Input: dimensioned drawing with shaded views. Units: mm. Origin: part minimum x, y, z. A direction names the side the tool comes from. Round coordinates to 2 decimals unless told otherwise and drop trailing zeros. Order: outer loops, then holes, each group sorted by start corner. A loop starts at its lowest first (then second) coordinate and runs counter-clockwise, first axis right, second up. Notation, with made-up numbers: M 26.5,1.25 L 39.5,1.25 A9 ccw 39.5,9.25 Z; hole C -27.75,11 d8. An arc over 180 degrees is marked long. Put each result on its own line as item: value. Start each with the question number.
1) Access query for the marked faces 1, 2 and 3. Directions: +Z, -Z, +X, -X, +Y, -Y. A direction counts if a zero-diameter tool reaches every point of the face in a straight line with its end or side. Return the directions, or none.
2) Material intervals for probe 1 along X at (y, z) = (2.25, 0.85); probe 2 along X at (y, z) = (3.5, 2.1); probe 3 along Y at (x, z) = (13.5, 0.95), sorted ascending. Write a range as [from, to].
3) First-contact query: P1, Ø1.5, axis at x = 39, z = 2, coming from the +Y side; P2, Ø1.5, axis at x = 40, y = 5, coming from the +Z side; P3, Ø1, axis at y = 13, z = 1.5, coming from the +X side; P4, Ø1, axis at y = 8.5, z = 2.5, coming from the +X side. Flat tips, straight axial feed; report the tip coordinate or a pass-through.
4) Section B-B, the plane x = 42. Return loops of the section in (y, z).
5) Section D-D, the plane x = 24.5. Return loops of the section in (y, z).
6) Section A-A, the plane y = 1.5. Return loops of the section in (x, z), then the cut area to 3 significant figures.
7) Section C-C, the plane y = 13. Return loops of the section in (x, z), then the cut area to 3 significant figures.
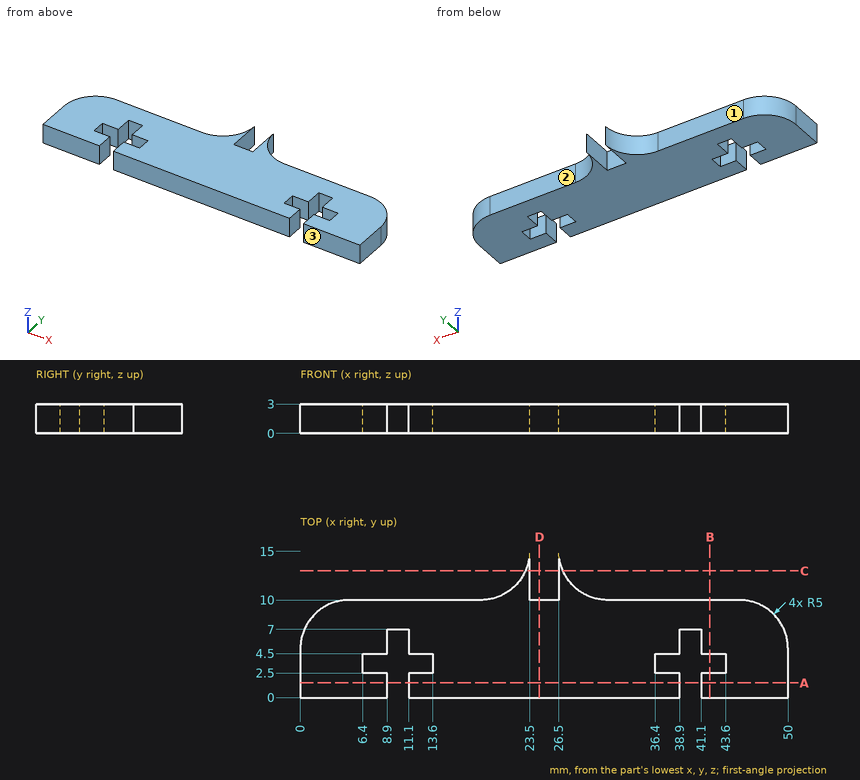
Result sheet:
1. face 1: +Z, -Z, -X, +Y
1. face 2: +Z, -Z, +X, +Y
1. face 3: +Z, -Z, +X, -X, -Y
2. probe 1: x = [0, 8.9], [11.1, 38.9], [41.1, 50]
2. probe 2: x = [0, 6.4], [13.6, 36.4], [43.6, 50]
2. probe 3: y = [0, 2.5], [4.5, 10]
3. P1: stops at y = 10
3. P2: passes through
3. P3: stops at x = 27.17
3. P4: stops at x = 49
4. outline: M 0,0 L 2.5,0 L 2.5,3 L 0,3 Z; M 4.5,0 L 10,0 L 10,3 L 4.5,3 Z
5. outline: M 0,0 L 10,0 L 10,3 L 0,3 Z
6. outline: M 0,0 L 8.9,0 L 8.9,3 L 0,3 Z; M 11.1,0 L 38.9,0 L 38.9,3 L 11.1,3 Z; M 41.1,0 L 50,0 L 50,3 L 41.1,3 Z
6. area: 137 mm2
7. outline: M 23.08,0 L 23.5,0 L 23.5,3 L 23.08,3 Z; M 26.5,0 L 26.92,0 L 26.92,3 L 26.5,3 Z
7. area: 2.50 mm2
